Can you work these out from the model? Positions are in its coordinate system, mm. Face numbers are marked on the shaded views. A direction names the side the tool comes from. Coordinates: 2 decimals unless noted, no trailing zeros. Write each loop counter-clockwise with the first axis right and the second up, starting at its lowest first coordinate (ties: lowest second). Pieces come first, ordered by that corner, then holes. Notation, with made-up numbers: (6, -7) -> (60, -7) arc R23 ccw to (60, 6) -> close; hole circle Ø1 at (49, -19). An arc over 180 degrees is marked (long way). Answer as CSV lines item,"result". Start each with the question number.
```python
from build123d import *

# Parameters (mm, degrees)
SKETCH1_R           = 26.67
BOSS_EXTRUDE1_DEPTH = 6.35
SHELL3_START        = 1.651
SHELL3_OUTLINE_R    = 26.67
SHELL3_DEPTH        = 3.048
BOSS_EXTRUDE3_START = -6.35
SKETCH7_R           = 24.892
SKETCH7_R_2         = 20.32
BOSS_EXTRUDE3_DEPTH = 6.35


# Read off the part's stored shape, not the designer's step: Shell3
with BuildPart() as part:
    # Sketch1 → Boss-Extrude1 (new body)
    with BuildSketch(Plane(origin=(0, 0, 0), x_dir=(1, 0, 0), z_dir=(0, 1, 0))):
        with Locations(Location((0, 0, 0), (0, 0, 270))):
            Circle(SKETCH1_R)
        Polygon((-5.19130268, 2.9972), (-6.921736907, 0), (-5.19130268, -2.9972), (-3.460868454, -5.9944), (3.460868454, -5.9944), (5.19130268, -2.9972), (6.921736907, 0), (5.19130268, 2.9972), (3.460868454, 5.9944), (-3.460868454, 5.9944), align=None, mode=Mode.SUBTRACT)
        with BuildLine():
            Line((-6.108033275, -6.459414023), (-16.189613398, -12.280017021))
            ThreePointArc((-16.189613398, -12.280017021), (0, -20.32), (16.189613398, -12.280017021))
            Line((16.189613398, -12.280017021), (6.108033275, -6.459414023))
            ThreePointArc((6.108033275, -6.459414023), (0, -8.89), (-6.108033275, -6.459414023))
        make_face(mode=Mode.SUBTRACT)
        with BuildLine():
            Line((-2.54, 8.519418994), (-2.54, 20.16062499))
            ThreePointArc((-2.54, 20.16062499), (-17.597636205, 10.16), (-18.729613398, -7.88060797))
            Line((-18.729613398, -7.88060797), (-8.648033275, -2.060004972))
            ThreePointArc((-8.648033275, -2.060004972), (-7.69896584, 4.445), (-2.54, 8.519418994))
        make_face(mode=Mode.SUBTRACT)
        with BuildLine():
            Line((8.648033275, -2.060004972), (18.729613398, -7.88060797))
            ThreePointArc((18.729613398, -7.88060797), (17.597636205, 10.16), (2.54, 20.16062499))
            Line((2.54, 20.16062499), (2.54, 8.519418994))
            ThreePointArc((2.54, 8.519418994), (7.69896584, 4.445), (8.648033275, -2.060004972))
        make_face(mode=Mode.SUBTRACT)
    extrude(amount=BOSS_EXTRUDE1_DEPTH)

    # Shell3 outline → Shell3 (cut)
    with BuildSketch(Plane(origin=(0, 0, 0), x_dir=(1, 0, 0), z_dir=(0, 1, 0)).offset(SHELL3_START)):
        Circle(SHELL3_OUTLINE_R)
        with BuildLine():
            ThreePointArc((0.889, 21.953007083), (19.027444147, 10.9855), (19.456361824, -10.206606958))
            Line((19.456361824, -10.206606958), (7.065610622, -3.052803416))
            Line((7.065610622, -3.052803416), (6.176610622, -4.592596584))
            Line((6.176610622, -4.592596584), (18.567361824, -11.746400126))
            ThreePointArc((18.567361824, -11.746400126), (0, -21.971), (-18.567361824, -11.746400126))
            Line((-18.567361824, -11.746400126), (-6.176610622, -4.592596584))
            Line((-6.176610622, -4.592596584), (-7.065610622, -3.052803416))
            Line((-7.065610622, -3.052803416), (-19.456361824, -10.206606958))
            ThreePointArc((-19.456361824, -10.206606958), (-19.027444147, 10.9855), (-0.889, 21.953007083))
            Line((-0.889, 21.953007083), (-0.889, 7.6454))
            Line((-0.889, 7.6454), (0.889, 7.6454))
            Line((0.889, 7.6454), (0.889, 21.953007083))
        make_face(mode=Mode.SUBTRACT)
    extrude(amount=SHELL3_DEPTH, mode=Mode.SUBTRACT)

    # Sketch7 → Boss-Extrude3 (add)
    with BuildSketch(Plane(origin=(0, 6.35, 0), x_dir=(1, 0, 0), z_dir=(0, 1, 0)).offset(BOSS_EXTRUDE3_START)):
        with Locations(Location((0, 0, 0), (0, 0, 270))):
            Circle(SKETCH7_R)
        Circle(SKETCH7_R_2, mode=Mode.SUBTRACT)
    extrude(amount=BOSS_EXTRUDE3_DEPTH)


solid = part.part
```
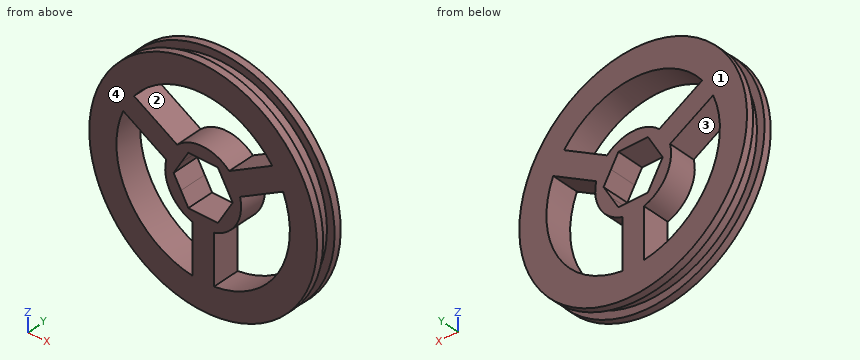
Q1. I need wall thicknesses on L1, parallel to Z at x = 0, y = 6; L2, parallel to X at y = 6, z = -15.5; L3, parallel to Z at x = 15.5, y = 2. Which ranges of each line are inside material? Lowest first, please.
Q2. Imagine slicing it at A-A (x = 0). Write out the boundary of the cut face in (y, z).
Q3. Imagine slicing it at C-C (z = 17.5). Write out the boundary of the cut face in (x, y).
Q4. If we mould it in two halves opening along X, with no side actions, what happens to the marked faces 3 and 4? For each: released by +X, released by -X, zero draft, split by the parting line, or undercut.
Q5. Imagine slicing it at D-D (x = 22.5). Write out the boundary of the cut face in (y, z), then the cut area to 3 significant figures.
Q6. Imagine slicing it at B-B (z = -10.5). Write out the boundary of the cut face in (x, y).
Q7. For pin 1 (6.5 mm diameter, centred on x = -11, z = 9, fed in from -Y); pin 2 (2.5 mm diameter, centred on y = 3, z = -12.5, fed in from +X); pin 3 (2 mm diameter, centred on x = -17.5, y = 5.5, fed in from +Z); pin 4 (0.9 mm diameter, centred on y = 2.5, z = -13, fed in from -X), each with a flat end and sliding along its axis, tell me the tip position at first contact or that it passes through.
Q8. Which directions (+Z, -Z, +X, -X, +Y, -Y) give clear straight access to the entire face, cutting with the end or side of a thin tool? Please do the marked faces 1 and 2.
Entries:
1,L1,"-26.67 to -5.99, 5.99 to 8.89, 20.32 to 26.67"
1,L2,"-21.7 to -13.14, -2.54 to 2.54, 13.14 to 21.7"
1,L3,"-19.48 to -13.14, 6.02 to 7.92, 9.98 to 11.88, 13.14 to 19.48"
2,outline,"(0, -26.67) -> (1.65, -26.67) -> (1.65, -24.89) -> (4.7, -24.89) -> (4.7, -26.67) -> (6.35, -26.67) -> (6.35, -5.99) -> (0, -5.99) -> close; (0, 5.99) -> (6.35, 5.99) -> (6.35, 8.89) -> (0, 8.89) -> close; (0, 20.32) -> (6.35, 20.32) -> (6.35, 26.67) -> (4.7, 26.67) -> (4.7, 24.89) -> (1.65, 24.89) -> (1.65, 26.67) -> (0, 26.67) -> close; hole (1.65, -20.32) -> (4.7, -20.32) -> (4.7, -7.65) -> (1.65, -7.65) -> close"
3,outline,"(-20.13, 0) -> (-10.33, 0) -> (-10.33, 6.35) -> (-20.13, 6.35) -> (-20.13, 4.7) -> (-17.7, 4.7) -> (-17.7, 1.65) -> (-20.13, 1.65) -> close; (10.33, 0) -> (20.13, 0) -> (20.13, 1.65) -> (17.7, 1.65) -> (17.7, 4.7) -> (20.13, 4.7) -> (20.13, 6.35) -> (10.33, 6.35) -> close"
4,face 3,"undercut"
4,face 4,"zero draft"
5,outline,"(0, -14.32) -> (1.65, -14.32) -> (1.65, -10.65) -> (4.7, -10.65) -> (4.7, -14.32) -> (6.35, -14.32) -> (6.35, 14.32) -> (4.7, 14.32) -> (4.7, 10.65) -> (1.65, 10.65) -> (1.65, 14.32) -> (0, 14.32) -> close"
5,area,"159 mm2"
6,outline,"(-24.52, 0) -> (-17.4, 0) -> (-17.4, 6.35) -> (-24.52, 6.35) -> (-24.52, 4.7) -> (-22.57, 4.7) -> (-22.57, 1.65) -> (-24.52, 1.65) -> close; (-2.54, 0) -> (2.54, 0) -> (2.54, 6.35) -> (-2.54, 6.35) -> close; (17.4, 0) -> (24.52, 0) -> (24.52, 1.65) -> (22.57, 1.65) -> (22.57, 4.7) -> (24.52, 4.7) -> (24.52, 6.35) -> (17.4, 6.35) -> close; hole (-0.89, 1.65) -> (0.89, 1.65) -> (0.89, 4.7) -> (-0.89, 4.7) -> close"
7,pin 1,"y = 0"
7,pin 2,"x = 22.2"
7,pin 3,"z = 20.95"
7,pin 4,"x = -21.5"
8,face 1,"+Z, -Z, +X, -X, +Y"
8,face 2,"+Y, -Y"
